Autodesk Inventor part; units mm, degrees
ref_plane "YZ Plane" through (0, 0, 0) normal (1, 0, 0) x (0, 1, 0)
ref_plane "XZ Plane" through (0, 0, 0) normal (0, 1, 0) x (-1, 0, 0)
ref_plane "XY Plane" through (0, 0, 0) normal (0, 0, 1) x (1, 0, 0)
sketch "WheelSketch" plane through (0, 0, 0) normal (0, 1, 0) x (-1, 0, 0)
  circle A0 centre (0, 0) radius 24.5
  dimension "EncoderWheel_Tyre_Diameter" = 49
extrude "Wheel" add sketch "WheelSketch" along normal blind 6
sketch "Sketch2" plane through (0, 6, 0) normal (0, 1, 0) x (1, 0, 0)
  circle A0 centre (0, 0) radius 24.5
  circle A1 centre (0, 0) radius 19.5
  dimension "EncoderWheel_Tyre_Thickness" = 5
extrude "Extrusion2" cut sketch "Sketch2" against normal blind 1.5 contours A1
sketch "Sketch3" plane through (0, 0, 0) normal (0, -1, 0) x (1, 0, 0)
  circle A0 centre (0, 0) radius 24.5
  circle A1 centre (0, 0) radius 19.5
  dimension "d7" = 5
extrude "Extrusion3" cut sketch "Sketch3" against normal blind 1.5 contours A1
sketch "InnerHoleSketch" plane through (0, 1.5, 0) normal (0, -1, 0) x (1, 0, 0)
  circle A0 centre (0, 0) radius 19.5
  circle A1 centre (0, 0) radius 6.25
  dimension "EncoderWheel_InnerHole_Diameter" = 12.5
extrude "InnerHole" cut sketch "InnerHoleSketch" against normal up to next contours A1
sketch "FasteningHoleSketch" plane through (0, 4.5, 0) normal (0, 1, 0) x (1, 0, 0)
  circle A0 centre (0, 0) radius 6.25
  circle A1 centre (0, 0) radius 19.5
  circle A2 centre (0, 9.5) radius 1.75
  line L0 (0, 0) -> (0, 29.2255) construction
  circle A3 centre (-6.7175, 6.7175) radius 1.75
  circle A4 centre (-9.5, 0) radius 1.75
  circle A5 centre (-6.7175, -6.7175) radius 1.75
  circle A6 centre (0, -9.5) radius 1.75
  circle A7 centre (6.7175, -6.7175) radius 1.75
  circle A8 centre (9.5, 0) radius 1.75
  circle A9 centre (6.7175, 6.7175) radius 1.75
  dimension "EncoderWheel_FasteningHole_Diameter" = 3.5
  dimension "EncoderWheel_FasteningHole_DistanceToCenter" = 9.5
  dimension "d17" = 360
extrude "FasteningHole" cut sketch "FasteningHoleSketch" against normal up to next contours A2 | A3 | A4 | A5 | A6 | A7 | A8 | A9
equation "\"d7\" = EncoderWheel_Tyre_Thickness"
equation "\"EncoderWheel_InnerDiameter\" = EncoderWheel_Tyre_Diameter - 2 * EncoderWheel_Tyre_Thickness"
properties part number "EncoderWheel" material "Rubber, Silicone"
Geometry: final body of the model. Coordinates: model frame, mm. A direction names the side the tool comes from. Round coordinates to 2 decimals unless told otherwise and drop trailing zeros. Loops run counter-clockwise (first coordinate to the right, second up) from the corner with the lowest first, then second, coordinate; pieces in that order, holes last. Notation, with made-up numbers: (-18.75, 30) -> (21.25, 30) arc R15 ccw to (21.25, 50) -> close; hole circle Ø11 at (45, -21). An arc over 180 degrees is marked (long way). Use one line per item in the form item = value. Start each with the question number.
1) Draft query along X for faces 4 (the cylindrical face through (-13.17, 2.96, -20.66)), 5 (the flat face through (16.45, 0, -10.77)), 6 (the cylindrical face through (11.169, 3.021, -0.526)). Return one class per face: released by +X, released by -X, zero draft, split by the parting line, or undercut.
2) Section B-B on z = -9.5. Output: boundary loops of the cut face in (x, y), then the cut area to 3 significant figures.
3) Section A-A on x = 0. Output: boundary loops of the cut face in (y, z), then the cut area to 4 significant figures.
4) Section D-D on z = 0. Output: boundary loops of the cut face in (x, y), then the cut area to 4 significant figures.
5) Access query for faces 1 (the flat face through (-5, 1.5, 5)), 2 (the cylindrical face through (5.96, 2.98, 1.88)), 3 (the flat face through (-5, 4.5, -5)). Directions: +Z, -Z, +X, -X, +Y, -Y. A direction counts if a zero-diameter tool reaches every point of the face in a straight line with its end or side. Return the directions, or none.
6) First-contact query: P1, Ø4.5, axis at x = 0, z = -9.5, coming from the +Y side; P2, Ø4, axis at x = -6.72, z = 6.72, coming from the -Y side; P3, Ø3, axis at y = 4, z = 15, coming from the -X side. Flat tips, straight axial feed; report the tip coordinate or a pass-through.
7) Line query: L1, parallel to Z at x = 0, y = 3.05; L2, parallel to Z at x = 0, y = 1; L3, parallel to Z at x = -1, y = 2.1. Output: solid intervals per line, ascending.
8) Section C-C on x = 9.5. Output: boundary loops of the cut face in (y, z).
Response:
q1.face_4 = split by the parting line
q1.face_5 = zero draft
q1.face_6 = undercut
q2.outline = (-22.58, 0) -> (-17.03, 0) -> (-17.03, 1.5) -> (-1.75, 1.5) -> (-1.75, 4.5) -> (-17.03, 4.5) -> (-17.03, 6) -> (-22.58, 6) -> close; (1.75, 1.5) -> (17.03, 1.5) -> (17.03, 0) -> (22.58, 0) -> (22.58, 6) -> (17.03, 6) -> (17.03, 4.5) -> (1.75, 4.5) -> close
q2.area = 158 mm^2
q3.outline = (0, -24.5) -> (6, -24.5) -> (6, -19.5) -> (4.5, -19.5) -> (4.5, -11.25) -> (1.5, -11.25) -> (1.5, -19.5) -> (0, -19.5) -> close; (0, 19.5) -> (1.5, 19.5) -> (1.5, 11.25) -> (4.5, 11.25) -> (4.5, 19.5) -> (6, 19.5) -> (6, 24.5) -> (0, 24.5) -> close; (1.5, -7.75) -> (4.5, -7.75) -> (4.5, -6.25) -> (1.5, -6.25) -> close; (1.5, 6.25) -> (4.5, 6.25) -> (4.5, 7.75) -> (1.5, 7.75) -> close
q3.area = 118.5 mm^2
q4.outline = (-24.5, 0) -> (-19.5, 0) -> (-19.5, 1.5) -> (-11.25, 1.5) -> (-11.25, 4.5) -> (-19.5, 4.5) -> (-19.5, 6) -> (-24.5, 6) -> close; (-7.75, 1.5) -> (-6.25, 1.5) -> (-6.25, 4.5) -> (-7.75, 4.5) -> close; (6.25, 1.5) -> (7.75, 1.5) -> (7.75, 4.5) -> (6.25, 4.5) -> close; (11.25, 1.5) -> (19.5, 1.5) -> (19.5, 0) -> (24.5, 0) -> (24.5, 6) -> (19.5, 6) -> (19.5, 4.5) -> (11.25, 4.5) -> close
q4.area = 118.5 mm^2
q5.face_1 = -Y
q5.face_2 = +Y, -Y
q5.face_3 = +Y
q6.P1 = 4.5
q6.P2 = 1.5
q6.P3 = -20.45
q7.L1 = -24.5 to -11.25, -7.75 to -6.25, 6.25 to 7.75, 11.25 to 24.5
q7.L2 = -24.5 to -19.5, 19.5 to 24.5
q7.L3 = -24.48 to -10.94, -8.06 to -6.17, 6.17 to 8.06, 10.94 to 24.48
q8.outline = (0, -22.58) -> (6, -22.58) -> (6, -17.03) -> (4.5, -17.03) -> (4.5, -1.75) -> (1.5, -1.75) -> (1.5, -17.03) -> (0, -17.03) -> close; (0, 17.03) -> (1.5, 17.03) -> (1.5, 1.75) -> (4.5, 1.75) -> (4.5, 17.03) -> (6, 17.03) -> (6, 22.58) -> (0, 22.58) -> close
